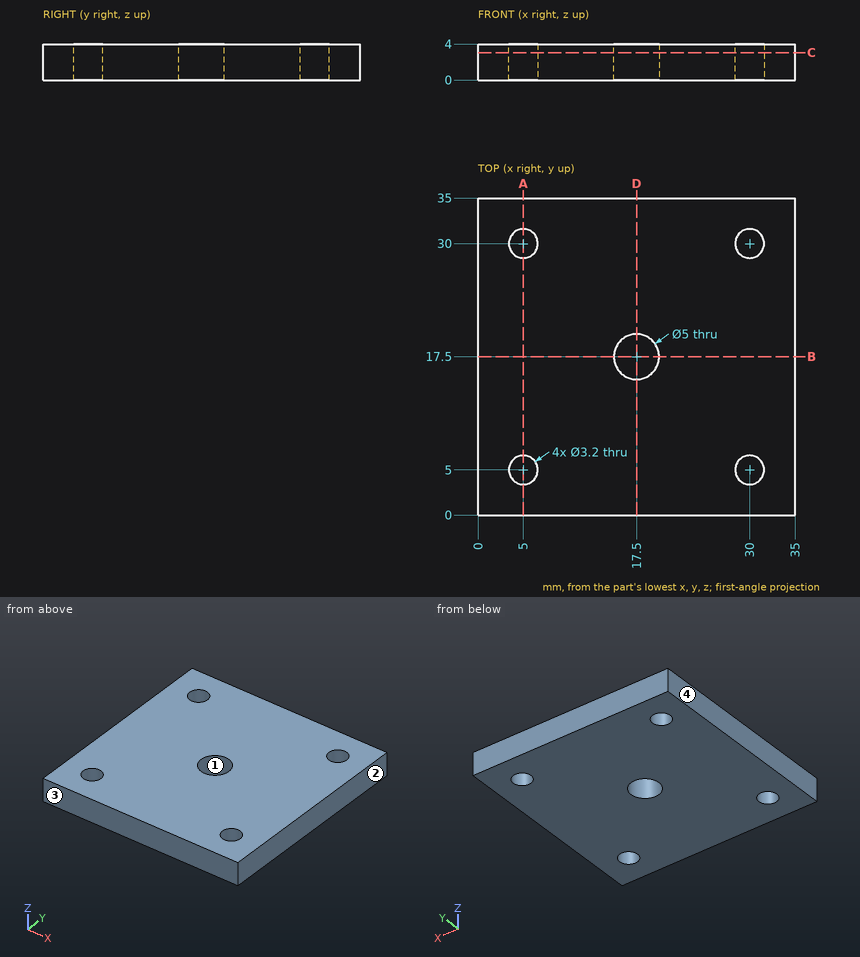
Input: dimensioned drawing with shaded views. Units: mm. Origin: part minimum x, y, z. Coordinates: 2 decimals unless noted, no trailing zeros. Order: outer loops, then holes, each group sorted by start corner. A loop starts at its lowest first (then second) coordinate and runs counter-clockwise, first axis right, second up.
(1) Material intervals for probe 1 along Y at (x, z) = (30, 1.95); probe 2 along Y at (x, z) = (17.5, 0.9); probe 3 along Y at (x, z) = (29, 2.25), sorted ascending.
(2) Section query C-C (z = 3.05). Return the cut outline in (x, y).
(3) Draft query along X for the marked faces 1, 2, 3 and 4. Return one class per face: pulls with the +X half, pulls with the -X half, needs draft (parallel to the pull), parting line crosses it, or undercut.
(4) Section query B-B (y = 17.5). Return the cut outline in (x, z), plus the area to 3 significant figures.
(5) Section query A-A (x = 5). Return the cut outline in (y, z), plus the area to 3 significant figures.
Solution:
1. probe 1: y = 0 to 3.4, 6.6 to 28.4, 31.6 to 35
1. probe 2: y = 0 to 15, 20 to 35
1. probe 3: y = 0 to 3.75, 6.25 to 28.75, 31.25 to 35
2. outline: (0, 0) - (35, 0) - (35, 35) - (0, 35) - close; hole circle Ø3.2 at (5, 5); hole circle Ø3.2 at (5, 30); hole circle Ø5 at (17.5, 17.5); hole circle Ø3.2 at (30, 5); hole circle Ø3.2 at (30, 30)
3. face 1: undercut
3. face 2: pulls with the +X half
3. face 3: needs draft
3. face 4: pulls with the -X half
4. outline: (0, 0) - (15, 0) - (15, 4) - (0, 4) - close; (20, 0) - (35, 0) - (35, 4) - (20, 4) - close
4. area: 120 mm2
5. outline: (0, 0) - (3.4, 0) - (3.4, 4) - (0, 4) - close; (6.6, 0) - (28.4, 0) - (28.4, 4) - (6.6, 4) - close; (31.6, 0) - (35, 0) - (35, 4) - (31.6, 4) - close
5. area: 114 mm2
